from build123d import *

# Parameters (mm, degrees)
SKIZZE1_W                       = 180
SKIZZE1_H                       = 25
AUFSATZ_LINEAR_AUSTRAGEN1_DEPTH = 1.5
SKIZZE2_W                       = 5
SKIZZE2_H                       = 5
AUFSATZ_LINEAR_AUSTRAGEN2_DEPTH = 5
SKIZZE3_R                       = 1.5
SCHNITT_LINEAR_AUSTRAGEN1_DEPTH = 5
SKIZZE4_W                       = 5
SKIZZE4_H                       = 5
AUFSATZ_LINEAR_AUSTRAGEN3_DEPTH = 5
SCHNITT_LINEAR_START            = -5
SKIZZE5_R                       = 1.5
SCHNITT_LINEAR_AUSTRAGEN2_DEPTH = 5


with BuildPart() as part:
    # Skizze1 → Aufsatz-Linear austragen1 (new body)
    with BuildSketch(Plane(origin=(0, 0, 0), x_dir=(1, 0, 0), z_dir=(0, 1, 0))):
        Rectangle(SKIZZE1_W, SKIZZE1_H)
    extrude(amount=AUFSATZ_LINEAR_AUSTRAGEN1_DEPTH)

    # Skizze2 → Aufsatz-Linear austragen2 (add)
    with BuildSketch(Plane(origin=(90, 0, 0), x_dir=(0, 0, -1), z_dir=(1, 0, 0))):
        with Locations((-10, 2.5)):
            Rectangle(SKIZZE2_W, SKIZZE2_H)
    extrude(amount=AUFSATZ_LINEAR_AUSTRAGEN2_DEPTH)

    # Skizze3 → Schnitt-Linear austragen1 (cut)
    with BuildSketch(Plane(origin=(95, 0, 0), x_dir=(0, 0, -1), z_dir=(1, 0, 0))):
        with Locations((-10, 2.5)):
            Circle(SKIZZE3_R)
    extrude(amount=-SCHNITT_LINEAR_AUSTRAGEN1_DEPTH, mode=Mode.SUBTRACT)

    # Skizze4 → Aufsatz-Linear austragen3 (add)
    with BuildSketch(Plane.ZY.offset(90)):
        with Locations((10, 2.5)):
            Rectangle(SKIZZE4_W, SKIZZE4_H)
    extrude(amount=AUFSATZ_LINEAR_AUSTRAGEN3_DEPTH)

    # Skizze5 → Schnitt-Linear austragen2 (cut)
    with BuildSketch(Plane.ZY.offset(95).offset(SCHNITT_LINEAR_START)):
        with Locations(Location((10, 2.5, 0), (0, 0, 180))):
            Circle(SKIZZE5_R)
    extrude(amount=SCHNITT_LINEAR_AUSTRAGEN2_DEPTH, mode=Mode.SUBTRACT)


solid = part.part
Work out the finished part from the listing and answer in its coordinate system (mm). A direction names the side the tool comes from. Round coordinates to 2 decimals unless told otherwise and drop trailing zeros. Order: outer loops, then holes, each group sorted by start corner. A loop starts at its lowest first (then second) coordinate and runs counter-clockwise, first axis right, second up. Notation, with made-up numbers: M -18,-28 L 36,-28 A23 cw 36,-5 Z; hole C -6.5,1.25 d8. An arc over 180 degrees is marked long. One line per item, written item: value.
Q1. Find section B-B on x = 27. Write down the section's boundary in (y, z), then the cut area to 3 significant figures.
Derived:
outline: M 0,-12.5 L 1.5,-12.5 L 1.5,12.5 L 0,12.5 Z
area: 37.5 mm²
Q2. Determine the mould class of faces 5 (the face through (-90, 4, 9)), 6 (the face through (-95, 4, 9)), 7 (the face through (95, 4, 11)) for opening direction X: released by +X, released by -X, zero draft, split by the parting line, or undercut.
Derived:
face 5: undercut
face 6: released by -X
face 7: released by +X
Q3. For faces 1 (the face through (-92.46, 1.49, 11.11)), 2 (the face through (90, 4, 11)), 3 (the face through (92.5, 1.6, 11.2)), 4 (the face through (92, 2, 7.5)), determine the directions among +Z, -Z, +X, -X, +Y, -Y from which every point of the face is accessible in a straight line to the end or side of a thin tool.
Derived:
face 1: -X
face 2: +Z, -Z, +Y
face 3: +X
face 4: -Z, +X, +Y, -Y
Q4. Straight lines are drawn through the part: line 1 (Y direction, x = 91.75, z = 10); line 2 (Z direction, x = -91.9, y = 2.5); line 3 (Y direction, x = -52.5, z = -8.5). For each, find the intervals that lie inside material, in ascending order.
Derived:
line 1: 0 to 1, 4 to 5
line 2: 7.5 to 8.5, 11.5 to 12.5
line 3: 0 to 1.5
Q5. Find section A-A on y = 2.5. Write down the section's boundary in (x, z).
Derived:
outline: M -95,7.5 L -90,7.5 L -90,8.5 L -95,8.5 Z; M -95,11.5 L -90,11.5 L -90,12.5 L -95,12.5 Z; M 90,7.5 L 95,7.5 L 95,8.5 L 90,8.5 Z; M 90,11.5 L 95,11.5 L 95,12.5 L 90,12.5 Z
Q6. Flat-ended cylindrical pins translate along their axes: pin 1 (6 mm diameter, centred on x = -36, z = 0, fed in from +Y); pin 2 (1.5 mm diameter, centred on x = 93.5, y = 2, fed in from -Z); pin 3 (3 mm diameter, centred on y = 3, z = 9.5, fed in from -X); pin 4 (1.1 mm diameter, centred on y = 3, z = 10.5, fed in from +X). Find the tip coordinate at first contact, or state that the pin passes through.
Derived:
pin 1: y = 1.5
pin 2: z = 7.5
pin 3: x = -95
pin 4: through
Q7. Find section C-C on z = -9. Write down the section's boundary in (x, y).
Derived:
outline: M -90,0 L 90,0 L 90,1.5 L -90,1.5 Z
